For this review, take the finished solid that the model builds, in its own axes (mm). Round coordinates to 2 decimals unless told otherwise and drop trailing zeros. Loops run counter-clockwise (first coordinate to the right, second up) from the corner with the lowest first, then second, coordinate; pieces in that order, holes last.
1. Consider section C-C on z = 1.1. State how many separate pieces and enclosed holes the cut face has, then the cut area to 3 significant figures.
2. To check wall thickness, follow line 1 along X through (y, z) = (-29, 0.3); line 2 along X through (y, z) = (-11, 5.45); line 3 along Y through (x, z) = (-15.5, 4.8). State the ranges of each line that lie inside material, in increasing order.
3. Consider section B-B on y = -1.5. State the section outline as (x, z) points.
4. Clearance check with flat-ended pins moving along their axes: pin 1 Ø1 at (y, z) = (88, 1.5) entering from +X; pin 2 Ø5 at (x, y) = (20.5, -12.5) entering from -Z; pin 3 Ø2 at (y, z) = (18.5, 5) entering from +X; pin 4 Ø4 at (x, y) = (-4.5, -23) entering from +Z. State where each tip first meets the part, or that it passes through.
5. Consider section A-A on x = -9.5. State the section outline as (y, z) points, then the cut area to 3 significant figures.
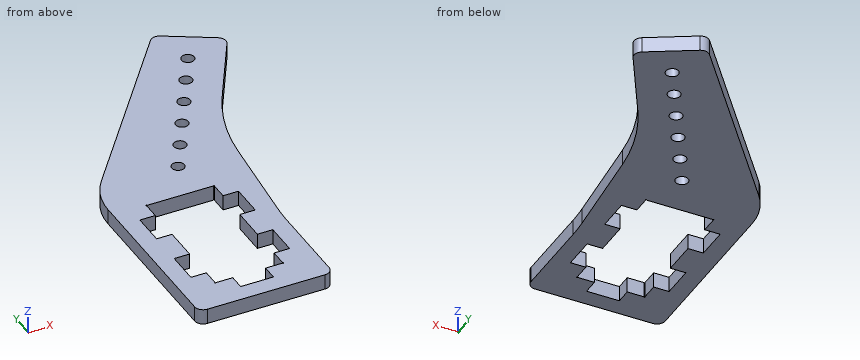
from build123d import *

# Parameters (mm, degrees)
SKETCH1_R           = 2.38125
BOSS_EXTRUDE1_DEPTH = 5.842
FILLET1_R           = 3.175
FILLET3_R           = 76.2
FILLET4_R           = 25.4
SKETCH2_R           = 0.1984375
CUT_EXTRUDE1_DEPTH  = 126.445308344


with BuildPart() as part:
    # Sketch1 → Boss-Extrude1 (new body)
    with BuildSketch(Plane.XY):
        Polygon((25.4, -38.1), (-25.4, -38.1), (-25.4, 38.1), (34.270606379, 113.488181024), (56.267651635, 100.788181024), (30.867651635, 56.794090512), (25.4, 0), align=None)
        with Locations((7.169129007, 41.147045256)):
            Circle(SKETCH1_R, mode=Mode.SUBTRACT)
        with Locations((13.519129007, 52.145567884)):
            Circle(SKETCH1_R, mode=Mode.SUBTRACT)
        with Locations((19.869129007, 63.144090512)):
            Circle(SKETCH1_R, mode=Mode.SUBTRACT)
        with Locations((26.219129007, 74.14261314)):
            Circle(SKETCH1_R, mode=Mode.SUBTRACT)
        with Locations((32.569129007, 85.141135768)):
            Circle(SKETCH1_R, mode=Mode.SUBTRACT)
        with Locations((38.919129007, 96.139658396)):
            Circle(SKETCH1_R, mode=Mode.SUBTRACT)
        Polygon((-12.800000054, -25.5), (-6.2, -25.5), (-6.2, -31.342), (6.2, -31.342), (6.2, -25.5), (12.800000054, -25.5), (12.800000054, -18.9), (18.642000054, -18.9), (18.642000054, -6.5), (12.800000054, -6.5), (12.800000054, 6.5), (18.642000054, 6.5), (18.642000054, 18.9), (12.800000054, 18.9), (12.800000054, 25.5), (-12.800000054, 25.5), (-12.800000054, 18.9), (-18.642000054, 18.9), (-18.642000054, 6.5), (-12.800000054, 6.5), (-12.800000054, -6.5), (-18.642000054, -6.5), (-18.642000054, -18.9), (-12.800000054, -18.9), align=None, mode=Mode.SUBTRACT)
    extrude(amount=BOSS_EXTRUDE1_DEPTH)

    # Fillet1
    fillet1_edges = [part.edges().sort_by_distance(p)[0] for p in [
        (34.270606379, 113.488181024, 2.921),
        (56.267651635, 100.788181024, 2.921),
        (25.4, -38.1, 2.921),
        (-25.4, -38.1, 2.921),
    ]]
    fillet(fillet1_edges, radius=FILLET1_R)

    # Fillet3
    # the kernel refuses this fillet: 76.2 mm, written as the material it adds along each edge
    with BuildSketch(Plane(origin=(30.867651635, 56.794090512, 0), x_dir=(-0.09582843425224026, -0.9953978657746682, 0), z_dir=(0, 0, 1))) as fillet3_piece_1:
        with BuildLine():
            CenterArc((FILLET3_R * 0.217130392833, FILLET3_R), FILLET3_R, 245.499003148, 24.500996852)
            Line((-FILLET3_R * 0.197578681587, FILLET3_R * 0.0900459442402), (0, 0))
            Line((0, 0), (FILLET3_R * 0.217130392833, 0))
        make_face()
    extrude(amount=5.842)
    with BuildSketch(Plane(origin=(25.4, 0, 0), x_dir=(0, -1, 0), z_dir=(0, 0, 1))) as fillet3_piece_2:
        with BuildLine():
            CenterArc((FILLET3_R * 0.048024725242, FILLET3_R), FILLET3_R, 264.500996852, 5.499003148)
            Line((-FILLET3_R * 0.0478037090103, FILLET3_R * 0.00460213422533), (0, 0))
            Line((0, 0), (FILLET3_R * 0.048024725242, 0))
        make_face()
    extrude(amount=5.842)

    # Fillet4
    fillet4_edges = [part.edges().sort_by_distance(p)[0] for p in [
        (-25.4, 38.1, 2.921),
    ]]
    fillet(fillet4_edges, radius=FILLET4_R)

    # Sketch2 → Cut-Extrude1 (cut, through all)
    with BuildSketch(Plane.XY.offset(5.842)):
        with Locations((-12.800000054, 25.5)):
            Circle(SKETCH2_R)
        with Locations((12.800000054, 25.5)):
            Circle(SKETCH2_R)
        with Locations((12.800000054, -25.5)):
            Circle(SKETCH2_R)
        with Locations((-12.800000054, -25.5)):
            Circle(SKETCH2_R)
    extrude(amount=-CUT_EXTRUDE1_DEPTH, mode=Mode.SUBTRACT)


solid = part.part
Resolved:
1. separate pieces: 1
1. enclosed holes: 7
1. area: 4,890 mm2
2. line 1: x = -25.4 to -6.2, 6.2 to 25.4
2. line 2: x = -25.4 to -18.64, 18.64 to 25.4
2. line 3: y = -38.1 to -18.9, -6.5 to 6.5, 18.9 to 50.61
3. outline: (-25.4, 0) - (-12.8, 0) - (-12.8, 5.84) - (-25.4, 5.84) - close; (12.8, 0) - (25.43, 0) - (25.43, 5.84) - (12.8, 5.84) - close
4. pin 1: stops at x = 49.17
4. pin 2: stops at z = 0
4. pin 3: stops at x = 27.28
4. pin 4: passes through
5. outline: (-38.1, 0) - (-25.5, 0) - (-25.5, 5.84) - (-38.1, 5.84) - close; (25.5, 0) - (58.19, 0) - (58.19, 5.84) - (25.5, 5.84) - close
5. area: 265 mm2
